Geometry: final body of the model. Coordinates: model frame, mm. Face numbers are marked on the shaded views. A direction names the side the tool comes from. Coordinates: 2 decimals unless noted, no trailing zeros. Order: outer loops, then holes, each group sorted by start corner. A loop starts at its lowest first (then second) coordinate and runs counter-clockwise, first axis right, second up. Notation, with made-up numbers: (4.5, -18) -> (36.5, -18) arc R13 ccw to (36.5, -6) -> close; hole circle Ø5 at (28.5, -16). An arc over 180 degrees is marked (long way). Use one line per item in the form item = value.
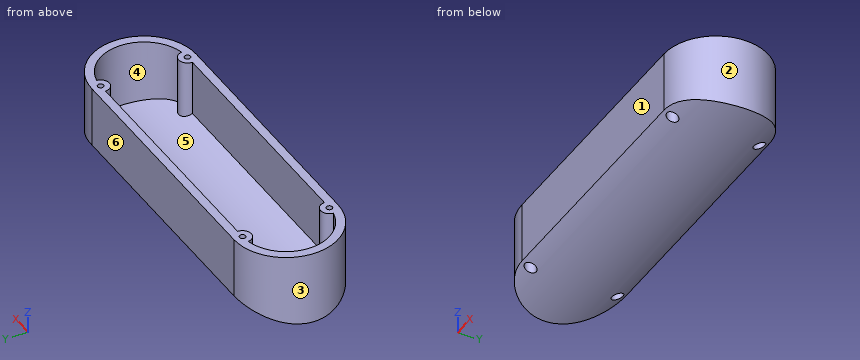
```python
from build123d import *

# Parameters (mm, degrees)
BOSS_EXTRUDE2_DEPTH                          = 45
CUT_EXTRUDE1_START                           = -120
CUT_EXTRUDE1_DEPTH                           = 207
CBORE_FOR_M3_HEX_SOCKET_HEAD_CAP_SCR_2_COUNT = 2
CBORE_FOR_M3_HEX_SOCKET_HEAD_CAP_SCR_2_PITCH = 145
CBORE_FOR_M3_HEX_SOCKET_HEAD_CAP_SCR_3_COUNT = 2
CBORE_FOR_M3_HEX_SOCKET_HEAD_CAP_SCR_3_PITCH = 153.248686781
CBORE_FOR_M3_HEX_SOCKET_HEAD_CAP_SCR_4_COUNT = 2
CBORE_FOR_M3_HEX_SOCKET_HEAD_CAP_SCR_4_PITCH = 49.6
CUT_EXTRUDE2_REACH                           = 227.539
CUT_EXTRUDE2_END_RADIUS                      = 58.5
CUT_EXTRUDE2_DIRECTION_2_DEPTH               = 226.538529612


with BuildPart() as part:
    # Sketch2 → Boss-Extrude2 (new body)
    with BuildSketch(Plane.XY):
        with BuildLine():
            Line((56.132610552, -127.487790866), (-88.867389448, -127.487790866))
            ThreePointArc((-88.867389448, -127.487790866), (-118.667389448, -157.287790866), (-88.867389448, -187.087790866))
            Line((-88.867389448, -187.087790866), (56.132610552, -187.087790866))
            ThreePointArc((56.132610552, -187.087790866), (85.932610552, -157.287790866), (56.132610552, -127.487790866))
        make_face()
    extrude(amount=-BOSS_EXTRUDE2_DEPTH)

    # Cut-Extrude1: read off the stored shape, not the designer's step
    # Cut-Extrude1 outline → Cut-Extrude1 (cut)
    with BuildSketch(Plane(origin=(0, 0, 0), x_dir=(0, 0, -1), z_dir=(1, 0, 0)).offset(CUT_EXTRUDE1_START)):
        with BuildLine():
            ThreePointArc((34.808748648, -127.487777676), (42.2355, -157.287790865), (34.808748648, -187.087804055))
            Line((34.808748648, -187.087804055), (45, -187.087790866))
            Line((45, -187.087790866), (45, -127.487790866))
            Line((45, -127.487790866), (34.808748648, -127.487777676))
        make_face()
    extrude(amount=CUT_EXTRUDE1_DEPTH, mode=Mode.SUBTRACT)

    # Sketch6 → CBORE for M3 Hex Socket Head Cap Screw1 (revolve, cut)
    with BuildSketch(Plane(origin=(56.132610552, -132.487790866, -40), x_dir=(0, 1, 0), z_dir=(1, 0, 0))):
        Polygon((0, 0), (0, 40), (1.7, 40), (1.7, 30), (3.25, 30), (3.25, 0.025), (3.275, 0), align=None)
    cbore_for_m3_hex_socket_head_cap_screw1 = revolve(axis=Axis((56.132610552, -132.487790866, -46.35), (0, 0, 1)), mode=Mode.SUBTRACT)

    # CBORE for M3 Hex Socket Head Cap Scr 2: CBORE for M3 Hex Socket Head Cap Screw1 ×2
    with Locations(*[(-i * CBORE_FOR_M3_HEX_SOCKET_HEAD_CAP_SCR_2_PITCH, 0, 0) for i in range(1, CBORE_FOR_M3_HEX_SOCKET_HEAD_CAP_SCR_2_COUNT)]):
        add(cbore_for_m3_hex_socket_head_cap_screw1, mode=Mode.SUBTRACT)

    # CBORE for M3 Hex Socket Head Cap Scr 3: CBORE for M3 Hex Socket Head Cap Screw1 ×2
    with Locations(*[Vector(-0.9461745026730805, -0.32365693332809825, 0) * (i * CBORE_FOR_M3_HEX_SOCKET_HEAD_CAP_SCR_3_PITCH) for i in range(1, CBORE_FOR_M3_HEX_SOCKET_HEAD_CAP_SCR_3_COUNT)]):
        add(cbore_for_m3_hex_socket_head_cap_screw1, mode=Mode.SUBTRACT)

    # CBORE for M3 Hex Socket Head Cap Scr 4: CBORE for M3 Hex Socket Head Cap Screw1 ×2
    with Locations(*[(0, -i * CBORE_FOR_M3_HEX_SOCKET_HEAD_CAP_SCR_4_PITCH, 0) for i in range(1, CBORE_FOR_M3_HEX_SOCKET_HEAD_CAP_SCR_4_COUNT)]):
        add(cbore_for_m3_hex_socket_head_cap_screw1, mode=Mode.SUBTRACT)

    # Cut-Extrude2: up to this cylinder (the profile starts inside it)
    cut_extrude2_end = Plane(origin=(-16.367389, -157.287790866, 21.2645), z_dir=(1, 0, 0)) * Cylinder(CUT_EXTRUDE2_END_RADIUS, 573.078, mode=Mode.PRIVATE)
    # Sketch7 → Cut-Extrude2 (cut, up to the surface)
    with BuildSketch(Plane.XY, mode=Mode.PRIVATE) as cut_extrude2_sk1:
        with BuildLine():
            ThreePointArc((-93.841919726, -181.583758608), (-88.615051766, -177.094162356), (-83.867389448, -182.087790866))
            Line((-83.867389448, -182.087790866), (51.132610552, -182.087790866))
            ThreePointArc((51.132610552, -182.087790866), (55.88027287, -177.094162356), (61.10714083, -181.583758608))
            ThreePointArc((61.10714083, -181.583758608), (80.932610552, -157.287790866), (61.10714083, -132.991823124))
            ThreePointArc((61.10714083, -132.991823124), (55.88027287, -137.481419376), (51.132610552, -132.487790866))
            Line((51.132610552, -132.487790866), (-83.867389448, -132.487790866))
            ThreePointArc((-83.867389448, -132.487790866), (-88.615051766, -137.481419376), (-93.841919726, -132.991823124))
            ThreePointArc((-93.841919726, -132.991823124), (-113.667389448, -157.287790866), (-93.841919726, -181.583758608))
        make_face()
    cut_extrude2_tool1 = extrude(cut_extrude2_sk1.sketch, amount=-CUT_EXTRUDE2_REACH, mode=Mode.PRIVATE) & cut_extrude2_end
    add(cut_extrude2_tool1.solids().sort_by_distance((-16.367389, -157.287791, 0))[0], mode=Mode.SUBTRACT)

    # Sketch7 → Cut-Extrude2 direction 2 (cut)
    with BuildSketch(Plane.XY):
        with BuildLine():
            ThreePointArc((-93.841919726, -181.583758608), (-88.615051766, -177.094162356), (-83.867389448, -182.087790866))
            Line((-83.867389448, -182.087790866), (51.132610552, -182.087790866))
            ThreePointArc((51.132610552, -182.087790866), (55.88027287, -177.094162356), (61.10714083, -181.583758608))
            ThreePointArc((61.10714083, -181.583758608), (80.932610552, -157.287790866), (61.10714083, -132.991823124))
            ThreePointArc((61.10714083, -132.991823124), (55.88027287, -137.481419376), (51.132610552, -132.487790866))
            Line((51.132610552, -132.487790866), (-83.867389448, -132.487790866))
            ThreePointArc((-83.867389448, -132.487790866), (-88.615051766, -137.481419376), (-93.841919726, -132.991823124))
            ThreePointArc((-93.841919726, -132.991823124), (-113.667389448, -157.287790866), (-93.841919726, -181.583758608))
        make_face()
    extrude(amount=CUT_EXTRUDE2_DIRECTION_2_DEPTH, mode=Mode.SUBTRACT)


solid = part.part
```
1) Section A-A, the plane z = -7. Output: boundary loops of the cut face in (x, y), and give its area (3 significant figures).
Results found:
outline = (-88.87, -187.09) -> (56.13, -187.09) arc R29.8 ccw to (56.13, -127.49) -> (-88.87, -127.49) arc R29.8 ccw to start; hole (-93.84, -181.58) arc R5 cw to (-83.87, -182.09) -> (51.13, -182.09) arc R5 cw to (61.11, -181.58) arc R24.8 ccw to (61.11, -132.99) arc R5 cw to (51.13, -132.49) -> (-83.87, -132.49) arc R5 cw to (-93.84, -132.99) arc R24.8 ccw to start; hole circle Ø3.4 at (-88.87, -182.09); hole circle Ø3.4 at (-88.87, -132.49); hole circle Ø3.4 at (56.13, -182.09); hole circle Ø3.4 at (56.13, -132.49)
area = 2,430 mm2
2) Section C-C, the plane y = -148. Output: boundary loops of the cut face in (x, z), and give its area (3 significant figures).
Results found:
outline = (-117.18, -41.55) -> (84.45, -41.55) -> (84.45, 0) -> (79.13, 0) -> (79.13, -36.49) -> (-111.86, -36.49) -> (-111.86, 0) -> (-117.18, 0) -> close
area = 1,410 mm2
3) Access query for the marked faces 5 and 6. Directions: +Z, -Z, +X, -X, +Y, -Y. A direction counts if a zero-diameter tool reaches every point of the face in a straight line with its end or side. Return the directions, or none.
Results found:
face_5 = +Z
face_6 = +Z, -Z, +X, -X, +Y
4) Section D-D, the plane z = -28.5. Output: boundary loops of the cut face in (x, y).
Results found:
outline = (-88.87, -187.09) -> (56.13, -187.09) arc R29.8 ccw to (56.13, -127.49) -> (-88.87, -127.49) arc R29.8 ccw to start; hole (-93.84, -181.58) arc R5 cw to (-83.87, -182.09) -> (51.13, -182.09) arc R5 cw to (61.11, -181.58) arc R24.8 ccw to (61.11, -132.99) arc R5 cw to (51.13, -132.49) -> (-83.87, -132.49) arc R5 cw to (-93.84, -132.99) arc R24.8 ccw to start; hole circle Ø6.5 at (-88.87, -182.09); hole circle Ø6.5 at (-88.87, -132.49); hole circle Ø6.5 at (56.13, -182.09); hole circle Ø6.5 at (56.13, -132.49)
5) Pull-direction query (X, two-part tool) for the marked faces 1, 2, 3 and 4; classes: released by +X, released by -X, zero draft, split by the parting line, or undercut.
Results found:
face_1 = zero draft
face_2 = released by +X
face_3 = released by -X
face_4 = undercut
6) Material intervals for probe 1 along Y at (x, z) = (9, -23); probe 2 along X at (y, z) = (-137, -23); probe 3 along Y at (x, z) = (58.5, -16), sorted ascending. Write a range as from..to.
Results found:
probe_1 = -187.09..-182.09, -132.49..-127.49
probe_2 = -110.7..-103.13, -91.02..-86.71, 53.98..58.29, 70.4..77.96
probe_3 = -186.99..-184.31, -179.86..-177.68, -136.89..-134.71, -130.26..-127.58
7) Contact query for flat-ended pins moving along their axis: P1, Ø2, axis at x = -49, y = -151.5, coming from the -Z side; P2, Ø5.5, axis at x = -88.87, y = -132.49, coming from the -Z side; P3, Ø1, axis at x = 64.5, z = -21, coming from the +Y side; P4, Ø3, axis at x = 56.13, y = -182.09, coming from the +Z side. Output: stop coordinate, or through.
Results found:
P1 = -42.05
P2 = -10
P3 = -128.55
P4 = through
8) Section B-B, the plane x = -15.5. Output: boundary loops of the cut face in (y, z).
Results found:
outline = (-187.09, -34.81) arc R63.5 ccw to (-127.49, -34.81) -> (-127.49, 0) -> (-132.49, 0) -> (-132.49, -31.72) arc R58.5 cw to (-182.09, -31.72) -> (-182.09, 0) -> (-187.09, 0) -> close
